Input: part model. Units: mm. Frame: model coordinates. A direction names the side the tool comes from. Coordinates: 2 decimals unless noted, no trailing zeros. Order: outer loops, then holes, each group sorted by start corner. A loop starts at its lowest first (then second) coordinate and runs counter-clockwise, first axis right, second up. Notation, with made-up numbers: M 48.25,26.25 L 84.25,26.25 A16 cw 84.25,36.25 Z; hole C 35,60 d3. An arc over 180 degrees is marked long. Answer in a Markdown table with one row per item.
from build123d import *

# Parameters (mm, degrees)
SKETCH1_W           = 12.6
SKETCH1_H           = 6.1
SKETCH1_R           = 0.9
BOSS_EXTRUDE1_DEPTH = 5.8
SKETCH2_W           = 1
SKETCH2_H           = 2.75
BOSS_EXTRUDE2_DEPTH = 1
SKETCH3_R           = 0.925
BOSS_EXTRUDE3_DEPTH = 15.75


with BuildPart() as part:
    # Sketch1 → Boss-Extrude1 (new body)
    with BuildSketch(Plane(origin=(0, 0, 0), x_dir=(1, 0, 0), z_dir=(0, 1, 0))):
        with Locations((6.3, 3.05)):
            Rectangle(SKETCH1_W, SKETCH1_H)
        with Locations(Location((3.04, 1.2, 0), (0, 0, 270))):
            Circle(SKETCH1_R, mode=Mode.SUBTRACT)
        with Locations(Location((9.74, 1.2, 0), (0, 0, 270))):
            Circle(SKETCH1_R, mode=Mode.SUBTRACT)
    extrude(amount=BOSS_EXTRUDE1_DEPTH)

    # Sketch2 → Boss-Extrude2 (add)
    with BuildSketch(Plane(origin=(0, 0, -6.1), x_dir=(-1, 0, 0), z_dir=(0, 0, -1))):
        with Locations((-4.5, 2.9)):
            Rectangle(SKETCH2_W, SKETCH2_H)
    extrude(amount=BOSS_EXTRUDE2_DEPTH)

    # Sketch3 → Boss-Extrude3 (add)
    with BuildSketch(Plane.XY):
        with Locations(Location((1.925, 2.9, 0), (0, 0, 180))):
            Circle(SKETCH3_R)
        with Locations(Location((6.555, 2.9, 0), (0, 0, 180))):
            Circle(SKETCH3_R)
    extrude(amount=BOSS_EXTRUDE3_DEPTH)


solid = part.part
1) Cut plane D-D, the plane x = 4.5. Output: boundary loops of the cut face in (y, z) (3 decimals), and give its area (3 significant figures).
Resolved:
| item | result |
|---|---|
| outline | M 0,-6.1 L 1.525,-6.1 L 1.525,-7.1 L 4.275,-7.1 L 4.275,-6.1 L 5.8,-6.1 L 5.8,0 L 0,0 Z |
| area | 38.1 mm2 |
2) Cut plane A-A, the plane x = 9.74. Output: boundary loops of the cut face in (y, z).
Resolved:
| item | result |
|---|---|
| outline | M 0,-6.1 L 5.8,-6.1 L 5.8,-2.1 L 0,-2.1 Z; M 0,-0.3 L 5.8,-0.3 L 5.8,0 L 0,0 Z |
3) Reachability of faces 1 (the face through (7.48, 2.86, 7.76)), 2 (the face through (6, 0, -3)), 3 (the face through (12.6, 3, -3)), 4 (the face through (4.5, 1.525, -6.6)), 5 (the face through (4, 2.9, -6.6)) from +Z, -Z, +X, -X, +Y, -Y: full face, straight path, thin tool, end or side. Return the list, or none.
Resolved:
| item | result |
|---|---|
| face 1 | +Z |
| face 2 | +Z, -Z, +X, -X, -Y |
| face 3 | +Z, -Z, +X, +Y, -Y |
| face 4 | -Z, +X, -X, -Y |
| face 5 | -Z, -X, +Y, -Y |
4) Cut plane B-B, the plane z = -1.2. Output: boundary loops of the cut face in (x, y), and give its area (3 significant figures).
Resolved:
| item | result |
|---|---|
| outline | M 0,0 L 2.14,0 L 2.14,5.8 L 0,5.8 Z; M 3.94,0 L 8.84,0 L 8.84,5.8 L 3.94,5.8 Z; M 10.64,0 L 12.6,0 L 12.6,5.8 L 10.64,5.8 Z |
| area | 52.2 mm2 |
5) Cut plane C-C, the plane y = 2.9. Output: boundary loops of the cut face in (x, z), and give its area (3 significant figures).
Resolved:
| item | result |
|---|---|
| outline | M 0,-6.1 L 4,-6.1 L 4,-7.1 L 5,-7.1 L 5,-6.1 L 12.6,-6.1 L 12.6,0 L 7.48,0 L 7.48,15.75 L 5.63,15.75 L 5.63,0 L 2.85,0 L 2.85,15.75 L 1,15.75 L 1,0 L 0,0 Z; hole C 3.04,-1.2 d1.8; hole C 9.74,-1.2 d1.8 |
| area | 131 mm2 |
6) Material intervals for probe 1 along X at (y, z) = (1.7, -1.2); probe 2 along X at (y, z) = (2.8, 14); probe 3 along Z at (x, y) = (9.75, 4.9), sorted ascending.
Resolved:
| item | result |
|---|---|
| probe 1 | x = 0 to 2.14, 3.94 to 8.84, 10.64 to 12.6 |
| probe 2 | x = 1.01 to 2.84, 5.64 to 7.47 |
| probe 3 | z = -6.1 to -2.1, -0.3 to 0 |
7) Mould query, pull axis X, two halves, no side actions, for faces 6 (the face through (4.5, 4.275, -6.6)), 7 (the face through (5, 2.9, -6.6)), 8 (the face through (10.63, 2.86, -1.32)). Classes: +X half, -X half, draft (parallel to the pull), parting line (faces both ways), or undercut.
Resolved:
| item | result |
|---|---|
| face 6 | draft |
| face 7 | +X half |
| face 8 | undercut |
8) Contact query for flat-ended pins moving along their axis: pin 1 (5 mm diameter, centred on x = 3.5, z = 7.5, fed in from -Y) (3 decimals); pin 2 (0.8 mm diameter, centred on x = 4.5, z = -7, fed in from -Y) (3 decimals); pin 3 (2 mm diameter, centred on x = 11, y = 1, fed in from -Z). Output: stop coordinate, or through.
Resolved:
| item | result |
|---|---|
| pin 1 | stops at y = 1.975 |
| pin 2 | stops at y = 1.525 |
| pin 3 | stops at z = -6.1 |
